Here's how the part is built. I have some questions about the finished solid (model axes, mm). Face numbers are marked on the shaded views. A direction names the side the tool comes from. Give positions to 0.01 mm unless a question says otherwise; leave off trailing zeros. Loops run counter-clockwise (first coordinate to the right, second up) from the corner with the lowest first, then second, coordinate; pieces in that order, holes last. Notation, with made-up numbers: (-37.75, -19) -> (14.25, -19) arc R18 ccw to (14.25, -14) -> close; hole circle Ø7 at (19.25, -34.75). An arc over 180 degrees is marked (long way). Answer in a Markdown table with one row per item. Add a question column.
Item 1: Which directions (+Z, -Z, +X, -X, +Y, -Y) give clear straight access to the entire face, cutting with the end or side of a thin tool? Please do the marked faces 1, 2 and 3.
Item 2: For P1, Ø22, axis at x = -3, y = 30, coming from the -Z side (3 decimals); P2, Ø10, axis at x = 16.5, z = -4, coming from the -Y side; P3, Ø6, axis at x = -14.605, z = 19.685, coming from the -Y side; P4, Ø6, axis at y = 49.5, z = 8.5, coming from the -X side (3 decimals), each with a flat end and sliding along its axis, tell me the tip position at first contact or that it passes through.
Item 3: If we section it at A-A (z = 0): Write out the boundary of the cut face in (x, y) (1 decimal), then the cut area to 3 significant figures.
Item 4: We'd pull the mould along Z, two halves only. Please class the marked faces 4, 5, 6 and 7: released by +Z, released by -Z, zero draft, split by the parting line, or undercut.
Item 5: If we section it at B-B (x = -9.5): Write out the boundary of the cut face in (y, z) (3 decimals), then the cut area to 3 significant figures.
Item 6: If I drill on line 1 (X direction, y = 55, z = 0) (1 decimal); line 2 (Z direction, x = 10.5, y = 33.5) (3 decimals); line 3 (Z direction, x = 15.24, y = 1.05) (1 decimal), over which ranges is the centre line in solid material (lowest first)?
Item 7: If we section it at D-D (x = 11.5): Write out the boundary of the cut face in (y, z) (3 decimals), then the cut area to 3 significant figures.
Item 8: If we section it at C-C (y = 23.5): Write out the boundary of the cut face in (x, z) (3 decimals), then the cut area to 3 significant figures.
Autodesk Inventor part; units mm, degrees
ref_plane "YZ Plane" through (0, 0, 0) normal (1, 0, 0) x (0, 1, 0)
ref_plane "XZ Plane" through (0, 0, 0) normal (0, 1, 0) x (-1, 0, 0)
ref_plane "XY Plane" through (0, 0, 0) normal (0, 0, 1) x (1, 0, 0)
sketch "Sketch1" plane through (0, 0, 0) normal (0, 1, 0) x (-1, 0, 0)
  line L0 (20.32, 10.16) -> (-20.32, 10.16)
  line L1 (-20.32, 10.16) -> (-20.32, -10.16)
  line L2 (-20.32, -10.16) -> (20.32, -10.16)
  line L3 (20.32, -10.16) -> (20.32, 10.16)
  line L4 (22.225, 12.065) -> (-22.225, 12.065)
  line L5 (-22.225, 12.065) -> (-22.225, -12.065)
  line L6 (-22.225, -12.065) -> (22.225, -12.065)
  line L7 (22.225, -12.065) -> (22.225, 12.065)
  point P0 (0, 0)
  dimension "d0" = 40.64
  dimension "d1" = 20.32
  dimension "d2" = 40.64
  dimension "d3" = 44.45
  dimension "d4" = 24.13
  dimension "d5" = 44.45
extrude "Extrusion1" add sketch "Sketch1" along normal blind 56.515
sketch "Sketch2" plane through (-20.32, 0, -10.16) normal (1, 0, 0) x (0, 0, -1)
  line L0 (0, 0) -> (-20.32, 0)
  line L1 (0, 0) -> (0, 56.515)
  line L2 (-20.32, 56.515) -> (0, 56.515)
  line L3 (-20.32, 0) -> (-20.32, 56.515)
  point P0 (-10.16, 0)
extrude "Extrusion2" cut sketch "Sketch2" against normal blind 56.515
sketch "Sketch3" plane through (20.32, 0, 10.16) normal (-1, 0, 0) x (0, 0, 1)
  line L0 (0, 0) -> (-20.32, 0)
  line L1 (0, 0) -> (0, 56.515)
  line L2 (-20.32, 56.515) -> (0, 56.515)
  line L3 (-20.32, 0) -> (-20.32, 56.515)
  point P0 (-10.16, 0)
extrude "Extrusion3" cut sketch "Sketch3" against normal blind 56.515
sketch "Sketch4" plane through (22.225, 0, 10.16) normal (0, 0, -1) x (-1, 0, 0)
  line L0 (44.45, 56.515) -> (44.45, 0)
  line L1 (0, 56.515) -> (44.45, 56.515)
  line L2 (0, 0) -> (0, 56.515)
  line L3 (44.45, 54.61) -> (0, 54.61)
  point P0 (22.225, 0)
extrude "Extrusion4" add sketch "Sketch4" along normal blind 20.32
sketch "Sketch5" plane through (-22.225, 0, 12.065) normal (0, 0, 1) x (1, 0, 0)
  line L0 (0, 0) -> (44.45, 0)
  line L1 (44.45, 0) -> (44.45, 56.515)
  line L2 (0, 0) -> (0, 56.515)
  line L3 (44.45, 1.905) -> (0, 1.905)
  point P0 (22.225, 0)
extrude "Extrusion5" add sketch "Sketch5" along normal blind 15.24
sketch "Sketch6" plane through (22.225, 0, -12.065) normal (0, 0, -1) x (-1, 0, 0)
  line L0 (0, 0) -> (44.45, 0)
  line L1 (44.45, 0) -> (44.45, 56.515)
  line L2 (0, 0) -> (0, 56.515)
  line L3 (44.45, 1.905) -> (0, 1.905)
  point P0 (22.225, 0)
extrude "Extrusion6" add sketch "Sketch6" along normal blind 15.24
sketch "Sketch7" plane through (0, 56.515, 0) normal (0, 1, 0) x (1, 0, 0)
  circle A0 centre (18.415, 0) radius 1.5875
  circle A1 centre (5.715, 0) radius 1.5875
  circle A2 centre (-12.065, 0) radius 3.175
  point P0 (0, 0)
  dimension "d18" = 3.175
  dimension "d19" = 3.175
  dimension "d20" = 6.35
extrude "Extrusion7" cut sketch "Sketch7" against normal blind 15.24
sketch "Sketch8" plane through (-22.225, 1.905, 12.065) normal (0, 1, 0) x (1, 0, 0)
  circle A0 centre (7.62, -7.62) radius 2.3495
  circle A1 centre (36.83, -7.62) radius 2.3495
  point P0 (22.225, 12.065)
  dimension "d23" = 4.699
  dimension "d24" = 4.699
extrude "Extrusion8" cut sketch "Sketch8" against normal blind 15.24
sketch "Sketch9" plane through (-22.225, 1.905, -12.065) normal (0, 1, 0) x (1, 0, 0)
  circle A0 centre (7.62, 7.62) radius 2.3495
  circle A1 centre (37.465, 7.62) radius 2.3495
  point P0 (22.225, -12.065)
  dimension "d27" = 4.699
  dimension "d28" = 4.699
extrude "Extrusion9" cut sketch "Sketch9" against normal blind 15.24
sketch "Sketch10" plane through (0, 56.515, 0) normal (0, 1, 0) x (1, 0, 0)
  circle A0 centre (-12.065, 0) radius 3.175
  line L0 (-22.225, 12.065) -> (-22.225, -12.065)
  line L1 (-22.225, -12.065) -> (22.225, -12.065)
  line L2 (22.225, 12.065) -> (-22.225, 12.065)
  line L3 (1.905, 12.065) -> (1.905, -12.065)
  point P0 (0, 0)
extrude "Extrusion10" cut sketch "Sketch10" against normal blind 19.05
fillet "Fillet1" radius 3.175 1 edges at (-22.225, 37.465, 11.1125)
fillet "Fillet2" radius 3.175 1 edges at (-22.225, 37.465, -11.1125)
fillet "Fillet3" radius 3.175 1 edges at (1.905, 37.465, 11.1125)
fillet "Fillet4" radius 3.175 1 edges at (1.905, 37.465, -11.1125)
properties part number "Autonomous - Ultrasonic Servo Mount"
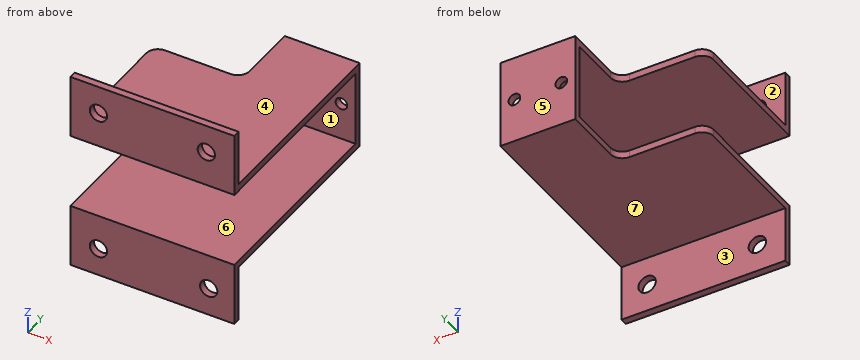
Recorded:
| question | item | result |
|---|---|---|
| 1 | face 1 | +X, -X, -Y |
| 1 | face 2 | +Z, +X, -X, +Y |
| 1 | face 3 | -Z, +X, -X, +Y |
| 2 | P1 | stops at z = -12.065 |
| 2 | P2 | stops at y = 54.61 |
| 2 | P3 | stops at y = 0 |
| 2 | P4 | stops at x = 1.905 |
| 3 | outline | (1.9, 54.6) -> (4.1, 54.6) -> (4.1, 56.5) -> (1.9, 56.5) -> close; (7.3, 54.6) -> (16.8, 54.6) -> (16.8, 56.5) -> (7.3, 56.5) -> close; (20, 54.6) -> (22.2, 54.6) -> (22.2, 56.5) -> (20, 56.5) -> close |
| 3 | area | 26.6 mm^2 |
| 4 | face 4 | released by +Z |
| 4 | face 5 | zero draft |
| 4 | face 6 | undercut |
| 4 | face 7 | released by -Z |
| 5 | outline | (0, -27.305) -> (1.905, -27.305) -> (1.905, -12.065) -> (37.465, -12.065) -> (37.465, -10.16) -> (0, -10.16) -> close; (0, 10.16) -> (37.465, 10.16) -> (37.465, 12.065) -> (1.905, 12.065) -> (1.905, 27.305) -> (0, 27.305) -> close |
| 5 | area | 201 mm^2 |
| 6 | line 1 | x = 1.9 to 4.1, 7.3 to 16.8, 20 to 22.2 |
| 6 | line 2 | z = -12.065 to -10.16, 10.16 to 12.065 |
| 6 | line 3 | z = -27.3 to -22, -17.3 to -10.2, 10.2 to 17.4, 21.9 to 27.3 |
| 7 | outline | (0, -27.305) -> (1.905, -27.305) -> (1.905, -12.065) -> (56.515, -12.065) -> (56.515, 12.065) -> (1.905, 12.065) -> (1.905, 27.305) -> (0, 27.305) -> (0, 10.16) -> (54.61, 10.16) -> (54.61, -10.16) -> (0, -10.16) -> close |
| 7 | area | 312 mm^2 |
| 8 | outline | (-22.225, -12.065) -> (22.225, -12.065) -> (22.225, -10.16) -> (-22.225, -10.16) -> close; (-22.225, 10.16) -> (22.225, 10.16) -> (22.225, 12.065) -> (-22.225, 12.065) -> close |
| 8 | area | 169 mm^2 |
